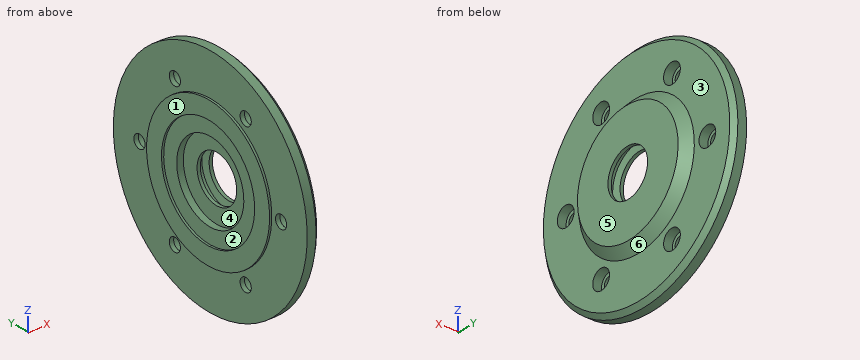
```python
from build123d import *

# Parameters (mm, degrees)
SKETCH_1_W                = 6
SKETCH_1_H                = 52
SKETCH_2_R                = 31
EXTRUDE_1_DEPTH           = 4
EXTRUDE_1_TAPER           = 45
SKETCH_3_R                = 33
EXTRUDE_2_DEPTH           = 1
HOLE_WIZARD_1_D           = 6
HOLE_WIZARD_1_DEPTH       = 7
HOLE_WIZARD_1_CBORE_D     = 9
HOLE_WIZARD_1_CBORE_DEPTH = 4
CHAMFER_1_SIZE            = 2


with BuildPart() as part:
    # Эскиз1 → Повернуть1 (revolve)
    with BuildSketch(Plane.XY, mode=Mode.PRIVATE) as revolve_1_sk:
        with Locations((3, 26)):
            Rectangle(SKETCH_1_W, SKETCH_1_H)
    revolve(revolve_1_sk.sketch.rotate(Axis((0, 0, 0), (1, 0, 0)), 270), axis=Axis((0, 0, 0), (1, 0, 0)))

    # Эскиз2 → Бобышка-Вытянуть1 (add)
    with BuildSketch(Plane(origin=(6, 0, 0), x_dir=(0, 0, -1), z_dir=(1, 0, 0))):
        Circle(SKETCH_2_R)
    extrude(amount=EXTRUDE_1_DEPTH, taper=EXTRUDE_1_TAPER)

    # Эскиз3 → Бобышка-Вытянуть2 (add)
    with BuildSketch(Plane.ZY):
        Circle(SKETCH_3_R)
    extrude(amount=EXTRUDE_2_DEPTH)

    # Эскиз4 → Вырез-Повернуть1 (revolve, cut)
    with BuildSketch(Plane.XY, mode=Mode.PRIVATE) as cut_revolve_1_sk:
        Polygon((-1, 25), (-1, 0), (10, 0), (10, 10.626409128), (8.5, 10.626409128), (8, 14), (5, 14), (4.5, 10.626409128), (3, 10.626409128), (3, 18), (0, 18), (0, 25), align=None)
    revolve(cut_revolve_1_sk.sketch.rotate(Axis((-1, 0, 0), (1, 0, 0)), 270), axis=Axis((-1, 0, 0), (1, 0, 0)), mode=Mode.SUBTRACT)

    # Отверстие1
    with Locations(Plane(origin=(6, 0, 0), x_dir=(0, 0, -1), z_dir=(1, 0, 0))):
        with Locations((32.908965344, -19), (0, -38), (-32.908965344, -19), (-32.908965344, 19), (0, 38), (32.908965344, 19)):
            CounterBoreHole(HOLE_WIZARD_1_D / 2, HOLE_WIZARD_1_CBORE_D / 2, HOLE_WIZARD_1_CBORE_DEPTH, depth=HOLE_WIZARD_1_DEPTH)

    # Фаска1
    chamfer_1_edges = [part.edges().sort_by_distance(p)[0] for p in [
        (6, 0, 52),
    ]]
    chamfer(chamfer_1_edges, length=CHAMFER_1_SIZE)


solid = part.part
```
Here's how the part is built. I have some questions about the finished solid (model axes, mm). Face numbers are marked on the shaded views. A direction names the side the tool comes from. Coordinates: 2 decimals unless noted, no trailing zeros. One line per question, with ' | ' between items. Start each with the question number.
1. Please list where these lines run through material, in increasing order: line 1 along Y through (x, z) = (1.1, 0); line 2 along Y through (x, z) = (5, -33); line 3 along Z through (x, y) = (4.25, 22). Write a range as [from, to].
2. I'm going to push flat-ended pins straight in: pin 1 Ø7 at (y, z) = (-38, 0) entering from +X; pin 2 Ø4.5 at (y, z) = (-39.5, -2) entering from +X; pin 3 Ø1.5 at (x, z) = (8, 20) entering from -Y. Where does each tip first touch, or does it pass through?
3. Which directions (+Z, -Z, +X, -X, +Y, -Y) give clear straight access to the entire face, cutting with the end or side of a thin tool? Please do the marked faces 1, 2 and 3.
4. If we mould it in two halves opening along Y, with no side actions, what happens to the marked faces 4, 5 and 6? For each: released by +Y, released by -Y, zero draft, split by the parting line, or undercut.
5. If we section it at A-A (y = -20.5): Give the number of separate pieces and of enclosed holes in the cut face, and give its area (3 significant figures).
Model answer:
1) line 1: y = [-52, -41], [-35, -18], [18, 35], [41, 52] | line 2: y = [-38.88, -23.5], [-14.5, 14.5], [23.5, 38.88] | line 3: z = [-46.84, -36.26], [-29.55, 29.55], [36.26, 46.84]
2) pin 1: stops at x = 2 | pin 2: stops at x = 6 | pin 3: stops at y = -22.23
3) face 1: +Z, -Z, -X, +Y, -Y | face 2: -X | face 3: +X
4) face 4: undercut | face 5: zero draft | face 6: split by the parting line
5) separate pieces: 3 | enclosed holes: 0 | area: 667 mm²
